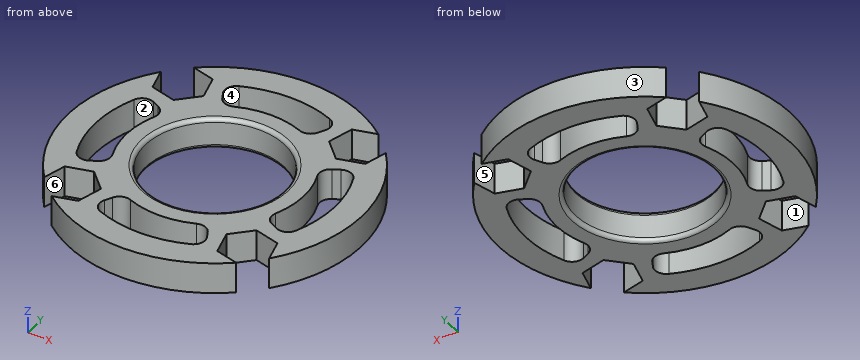
```python
from build123d import *

# Parameters (mm, degrees)
SKETCH1_R           = 19
SKETCH1_R_2         = 9
BOSS_EXTRUDE1_DEPTH = 4
CUT_EXTRUDE1_DEPTH  = 4
FILLET1_R           = 0.5


with BuildPart() as part:
    # Sketch1 → Boss-Extrude1 (new body)
    with BuildSketch(Plane.XY):
        Circle(SKETCH1_R)
        Circle(SKETCH1_R_2, mode=Mode.SUBTRACT)
        with BuildLine():
            Line((6.689691504, 12.241024694), (6.226047976, 11.350373764))
            ThreePointArc((6.226047976, 11.350373764), (5.41320923, 10.635157913), (4.330662681, 10.653420143))
            ThreePointArc((4.330662681, 10.653420143), (0, 11.5), (-4.330662681, 10.653420143))
            ThreePointArc((-4.330662681, 10.653420143), (-5.41320923, 10.635157913), (-6.226047976, 11.350373764))
            Line((-6.226047976, 11.350373764), (-6.689691504, 12.241024694))
            ThreePointArc((-6.689691504, 12.241024694), (-6.768746058, 13.446590252), (-5.933372603, 14.319395572))
            ThreePointArc((-5.933372603, 14.319395572), (0, 15.5), (5.933372603, 14.319395572))
            ThreePointArc((5.933372603, 14.319395572), (6.768746058, 13.446590252), (6.689691504, 12.241024694))
        make_face(mode=Mode.SUBTRACT)
        with BuildLine():
            Line((12.241024694, 6.689691504), (11.350373764, 6.226047976))
            ThreePointArc((11.350373764, 6.226047976), (10.635157913, 5.41320923), (10.653420143, 4.330662681))
            ThreePointArc((10.653420143, 4.330662681), (11.5, 0), (10.653420143, -4.330662681))
            ThreePointArc((10.653420143, -4.330662681), (10.635157913, -5.41320923), (11.350373764, -6.226047976))
            Line((11.350373764, -6.226047976), (12.241024694, -6.689691504))
            ThreePointArc((12.241024694, -6.689691504), (13.446590252, -6.768746058), (14.319395572, -5.933372603))
            ThreePointArc((14.319395572, -5.933372603), (15.5, 0), (14.319395572, 5.933372603))
            ThreePointArc((14.319395572, 5.933372603), (13.446590252, 6.768746058), (12.241024694, 6.689691504))
        make_face(mode=Mode.SUBTRACT)
        with BuildLine():
            Line((6.689691504, -12.241024694), (6.226047976, -11.350373764))
            ThreePointArc((6.226047976, -11.350373764), (5.41320923, -10.635157913), (4.330662681, -10.653420143))
            ThreePointArc((4.330662681, -10.653420143), (0, -11.5), (-4.330662681, -10.653420143))
            ThreePointArc((-4.330662681, -10.653420143), (-5.41320923, -10.635157913), (-6.226047976, -11.350373764))
            Line((-6.226047976, -11.350373764), (-6.689691504, -12.241024694))
            ThreePointArc((-6.689691504, -12.241024694), (-6.768746058, -13.446590252), (-5.933372603, -14.319395572))
            ThreePointArc((-5.933372603, -14.319395572), (0, -15.5), (5.933372603, -14.319395572))
            ThreePointArc((5.933372603, -14.319395572), (6.768746058, -13.446590252), (6.689691504, -12.241024694))
        make_face(mode=Mode.SUBTRACT)
        with BuildLine():
            Line((-12.241024694, -6.689691504), (-11.350373764, -6.226047976))
            ThreePointArc((-11.350373764, -6.226047976), (-10.635157913, -5.41320923), (-10.653420143, -4.330662681))
            ThreePointArc((-10.653420143, -4.330662681), (-11.5, 0), (-10.653420143, 4.330662681))
            ThreePointArc((-10.653420143, 4.330662681), (-10.635157913, 5.41320923), (-11.350373764, 6.226047976))
            Line((-11.350373764, 6.226047976), (-12.241024694, 6.689691504))
            ThreePointArc((-12.241024694, 6.689691504), (-13.446590252, 6.768746058), (-14.319395572, 5.933372603))
            ThreePointArc((-14.319395572, 5.933372603), (-15.5, 0), (-14.319395572, -5.933372603))
            ThreePointArc((-14.319395572, -5.933372603), (-13.446590252, -6.768746058), (-12.241024694, -6.689691504))
        make_face(mode=Mode.SUBTRACT)
    extrude(amount=BOSS_EXTRUDE1_DEPTH)

    # Sketch2 → Cut-Extrude1 (cut)
    with BuildSketch(Plane(origin=(0, 0, 0), x_dir=(-1, 0, 0), z_dir=(0, 0, -1))):
        Polygon((10.608852647, -8.200187733), (8.200187733, -10.608852647), (9.081820281, -13.899150108), (12.372117742, -14.780782656), (14.780782656, -12.372117742), (13.899150108, -9.081820281), align=None)
        Polygon((13.899150108, 9.081820281), (14.780782656, 12.372117742), (12.372117742, 14.780782656), (9.081820281, 13.899150108), (8.200187733, 10.608852647), (10.608852647, 8.200187733), align=None)
        Polygon((-8.200187733, -10.608852647), (-10.608852647, -8.200187733), (-13.899150108, -9.081820281), (-14.780782656, -12.372117742), (-12.372117742, -14.780782656), (-9.081820281, -13.899150108), align=None)
        Polygon((-10.608852647, 8.200187733), (-8.200187733, 10.608852647), (-9.081820281, 13.899150108), (-12.372117742, 14.780782656), (-14.780782656, 12.372117742), (-13.899150108, 9.081820281), align=None)
    extrude(amount=-CUT_EXTRUDE1_DEPTH, mode=Mode.SUBTRACT)

    # Fillet1
    fillet1_edges = [part.edges().sort_by_distance(p)[0] for p in [
        (-9, 0, 0),
        (-9, 0, 4),
    ]]
    fillet(fillet1_edges, radius=FILLET1_R)


solid = part.part
```
Could you check a few things on this model? Use its own coordinates, in mm. Face numbers are marked on the shaded views. A direction names the side the tool comes from. Round coordinates to 2 decimals unless told otherwise and drop trailing zeros. Order: outer loops, then holes, each group sorted by start corner. A loop starts at its lowest first (then second) coordinate and runs counter-clockwise, first axis right, second up. Notation, with made-up numbers: M 32.5,84 L 86.5,84 A14 ccw 86.5,105 Z; hole C -19,-9.75 d2. An arc over 180 degrees is marked long. One line per question, with ' | ' between items. Start each with the question number.
(1) Suppose I cut it at C-C on z = 2.4. Count the separate pieces of the cut face and the enclosed holes in it, then the cut area to 3 significant figures.
(2) Suppose I cut it at A-A on y = 0. List the corners of the cut face in (x, z) for me.
(3) For the marked faces 4, 5 and 6, which set-ups out of +Z, -Z, +X, -X, +Y, -Y let a thin tool reach every point of the face, with its end or its side?
(4) Please list where these lines run through material, in increasing order: line 1 along Y through (x, z) = (-5.5, 1.1); line 2 along Y through (x, z) = (-5, 3.35); line 3 along X through (y, z) = (-3.5, 2.8).
(5) Thinking about a two-plate mould opening in X: for the marked faces 1, 2 and 3, which applies, +X half, -X half, draft (parallel to the pull), parting line (faces both ways), or undercut?
(6) For P1, Ø2, axis at y = -2, z = 3, coming from the +X side, with a flat end and sliding along its axis, tell me the tip position at first contact or that it passes through.
Geometry results:
1) separate pieces: 1 | enclosed holes: 5 | area: 554 mm²
2) outline: M -19,0 L -15.5,0 L -15.5,4 L -19,4 Z; M -11.5,0 L -9.5,0 A0.5 ccw -9,0.5 L -9,3.5 A0.5 ccw -9.5,4 L -11.5,4 Z; M 9,0.5 A0.5 ccw 9.5,0 L 11.5,0 L 11.5,4 L 9.5,4 A0.5 ccw 9,3.5 Z; M 15.5,0 L 19,0 L 19,4 L 15.5,4 Z
3) face 4: +Z, -Z | face 5: +Z, -Z, +Y | face 6: +Z, -Z, -Y
4) line 1: -18.19 to -14.49, -10.67 to -7.12, 7.12 to 10.67, 14.49 to 18.19 | line 2: -18.33 to -14.67, -10.55 to -7.48, 7.48 to 10.55, 14.67 to 18.33 | line 3: -18.67 to -15.1, -10.95 to -8.29, 8.29 to 10.95, 15.1 to 18.67
5) face 1: -X half | face 2: undercut | face 3: parting line
6) P1: x = 18.97
